```python
from build123d import *

# Parameters (mm, degrees)
F2_DEPTH = 30
F3_DEPTH = 30
F4_R     = 7.5
F4_R_2   = 6
F5_DEPTH = 25


with BuildPart() as f2:
    # F0 (on Front) → F2 (new body)
    with BuildSketch(Plane.XZ):
        Polygon((0, 0), (0, -13), (10, -13), (10, -3), (52, -3), (52, -13), (62, -13), (62, 0), align=None)
    extrude(amount=F2_DEPTH)

    # F1 (on face) → F3 (join)
    with BuildSketch(Plane.XZ):
        Polygon((62, 0), (0, 0), (0, -13), (10, -13), (10, -3), (52, -3), (52, -13), (62, -13), align=None)
    extrude(amount=F3_DEPTH)

    # F4 (on face) → F5 (cut)
    with BuildSketch(Plane.XY):
        with Locations((14.728305, -15.297354)):
            Circle(F4_R)
        with Locations((43.501947, -15.963921)):
            Circle(F4_R_2)
    extrude(amount=-F5_DEPTH, mode=Mode.SUBTRACT)


solid = f2.part
```
CAD build for the part. Positions are in the model's coordinates, mm. A direction names the side the tool comes from. Coordinates: 2 decimals unless noted, no trailing zeros. Order: outer loops, then holes, each group sorted by start corner. A loop starts at its lowest first (then second) coordinate and runs counter-clockwise, first axis right, second up. Notation, with made-up numbers: (89.5, 1.5) - (123.5, 1.5) arc R20 ccw to (123.5, 28.5) - close; hole circle Ø2 at (86.5, 1.5). An arc over 180 degrees is marked (long way). Answer in a Markdown table with one row per item.
1. Slice it at A-A, the plane z = -8. List the corners of the cut face in (x, y), then the cut area to 3 significant figures.
Answer:
| item | result |
|---|---|
| outline | (0, -30) - (10, -30) - (10, -21.12) arc R7.5 cw to (10, -9.48) - (10, 0) - (0, 0) - close; (52, -30) - (62, -30) - (62, 0) - (52, 0) - close |
| area | 578 mm² |
2. Slice it at B-B, the plane x = 15. List the corners of the cut face in (y, z), then the cut area to 3 significant figures.
Answer:
| item | result |
|---|---|
| outline | (-30, -3) - (-22.79, -3) - (-22.79, 0) - (-30, 0) - close; (-7.8, -3) - (0, -3) - (0, 0) - (-7.8, 0) - close |
| area | 45.0 mm² |
3. Drill centre lines: L1, parallel to Y at x = 15, z = -1.75; L2, parallel to X at y = -5.5, z = -10.5; L3, parallel to Z at x = 32, y = -20.75. Where is each one in solid material? Low to high. Write a range as from..to.
Answer:
| item | result |
|---|---|
| L1 | -30..-22.79, -7.8..0 |
| L2 | 0..10, 52..62 |
| L3 | -3..0 |
4. Flat gauge pin, fed straight in: P1, Ø3, axis at x = 12.5, y = -22.5, coming from the -Z side. Where does the tip first touch, or does it go through?
Answer:
| item | result |
|---|---|
| P1 | z = -3 |
5. Slice it at C-C, the plane y = -4.25. List the corners of the cut face in (x, z), then the cut area to 3 significant figures.
Answer:
| item | result |
|---|---|
| outline | (0, -13) - (10, -13) - (10, -3) - (52, -3) - (52, -13) - (62, -13) - (62, 0) - (0, 0) - close |
| area | 386 mm² |
6. Pull direction Y, two halves, no side cores. Call faces 1 (the face through (46.728, -10.905, -1.479)), 2 (the face through (10, -25, -8)), 3 (the face through (24, -30, -2)): +Y half, -Y half, draft (parallel to the pull), parting line (faces both ways), or undercut.
Answer:
| item | result |
|---|---|
| face 1 | undercut |
| face 2 | draft |
| face 3 | -Y half |
7. 3-axis set-ups, long thin cutter, end or side, ignore diameter. For faces 4 (the face through (0, -15, -6)), 5 (the face through (10, -5, -8)): which of +Z, -Z, +X, -X, +Y, -Y reach the whole face in a straight line?
Answer:
| item | result |
|---|---|
| face 4 | +Z, -Z, -X, +Y, -Y |
| face 5 | -Z, +Y, -Y |
8. Slice it at D-D, the plane y = -13.5. List the corners of the cut face in (x, z).
Answer:
| item | result |
|---|---|
| outline | (0, -13) - (7.45, -13) - (7.45, 0) - (0, 0) - close; (22.01, -3) - (38.03, -3) - (38.03, 0) - (22.01, 0) - close; (48.97, -3) - (52, -3) - (52, -13) - (62, -13) - (62, 0) - (48.97, 0) - close |
